Here's how the part is built. I have some questions about the finished solid (model axes, mm). Coordinates: 2 decimals unless noted, no trailing zeros. Write each loop counter-clockwise with the first axis right and the second up, starting at its lowest first coordinate (ties: lowest second). Pieces come first, ordered by that corner, then holes.
Item 1: I want a section at B-B (z = 0). Please give me the cut outline in (x, y).
Item 2: I want a section at C-C (x = -11.5). Please give me the cut outline in (y, z).
Item 3: Please list where these lines run through material, in increasing order: line 1 (X direction, y = -0.7, z = 20.5); line 2 (Z direction, x = -23.5, y = -0.15); line 3 (Z direction, x = 6, y = -0.4).
Item 4: I want a section at D-D (y = -1.05). Please give me the cut outline in (x, z).
Item 5: I want a section at A-A (x = 0). Please give me the cut outline in (y, z), and give its area (3 significant figures).
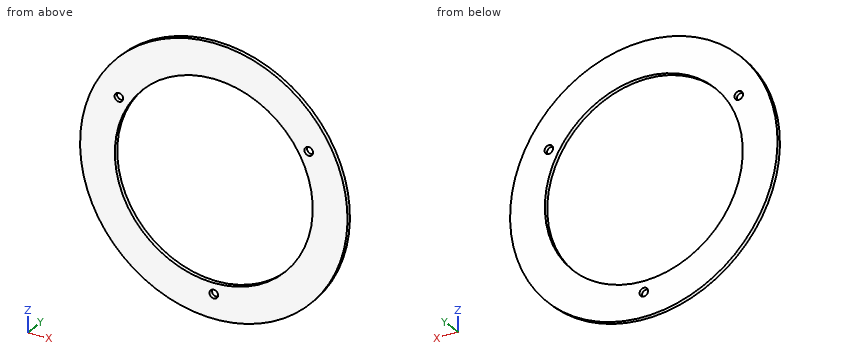
from build123d import *

# Parameters (mm, degrees)
SKETCH1_R          = 50
SKETCH1_R_2        = 37
BASE_FLANGE1_DEPTH = 1.5
SKETCH6_R          = 1.6
CUT_EXTRUDE1_DEPTH = 71.726586232


# Sheet-metal steps are written as plain solids
with BuildPart() as part:
    # Sketch1 → Base-Flange1 (new body)
    with BuildSketch(Plane(origin=(0, 0, 0), x_dir=(1, 0, 0), z_dir=(0, 1, 0))):
        with Locations(Location((0, 0, 0), (0, 0, 270))):
            Circle(SKETCH1_R)
        with Locations(Location((0, 0, 0), (0, 0, 270))):
            Circle(SKETCH1_R_2, mode=Mode.SUBTRACT)
    extrude(amount=-BASE_FLANGE1_DEPTH)

    # Sketch6 → Cut-Extrude1 (cut, through all)
    with BuildSketch(Plane(origin=(0, 0, 0), x_dir=(1, 0, 0), z_dir=(0, 1, 0))):
        with Locations(Location((0, 41, 0), (0, 0, 270))):
            Circle(SKETCH6_R)
        with Locations(Location((35.507041555, -20.5, 0), (0, 0, 270))):
            Circle(SKETCH6_R)
        with Locations(Location((-35.507041555, -20.5, 0), (0, 0, 270))):
            Circle(SKETCH6_R)
    extrude(amount=-CUT_EXTRUDE1_DEPTH, mode=Mode.SUBTRACT)


solid = part.part
Answer:
1. outline: (-50, -1.5) - (-37, -1.5) - (-37, 0) - (-50, 0) - close; (37, -1.5) - (50, -1.5) - (50, 0) - (37, 0) - close
2. outline: (-1.5, -48.66) - (0, -48.66) - (0, -35.17) - (-1.5, -35.17) - close; (-1.5, 35.17) - (0, 35.17) - (0, 48.66) - (-1.5, 48.66) - close
3. line 1: x = -45.6 to -37.11, -33.91 to -30.8, 30.8 to 33.91, 37.11 to 45.6
3. line 2: z = -44.13 to -28.58, 28.58 to 44.13
3. line 3: z = -49.64 to -36.51, 36.51 to 49.64
4. outline: circle Ø100 at (0, 0); hole circle Ø3.2 at (-35.51, 20.5); hole circle Ø74 at (0, 0); hole circle Ø3.2 at (0, -41); hole circle Ø3.2 at (35.51, 20.5)
5. outline: (-1.5, -50) - (0, -50) - (0, -42.6) - (-1.5, -42.6) - close; (-1.5, -39.4) - (0, -39.4) - (0, -37) - (-1.5, -37) - close; (-1.5, 37) - (0, 37) - (0, 50) - (-1.5, 50) - close
5. area: 34.2 mm2
